The model under review builds one solid part; all positions refer to its coordinate system, in mm. Face numbers are marked on the shaded views. A direction names the side the tool comes from. Coordinates: 2 decimals unless noted, no trailing zeros. Loops run counter-clockwise (first coordinate to the right, second up) from the corner with the lowest first, then second, coordinate; pieces in that order, holes last. Notation, with made-up numbers: (72, -1) - (100, -1) arc R10 cw to (100, 6) - close; hole circle Ø1 at (-1, 84). An arc over 180 degrees is marked (long way). One line per item, written item: value. Start each with the question number.
1. Insertion check: P1, Ø4, axis at x = 45.5, z = 23, coming from the +Y side; P2, Ø1.3, axis at y = 15, z = 20, coming from the -X side; P3, Ø1.3, axis at x = 66, z = 38, coming from the +Y side. Each pin has a flat end and moves straight along its axis. Give the tip position at first contact, or say it passes through.
2. We need section D-D, the plane x = 37. Give the boundary of the cut face in (y, z) (3 decimals), then the cut area to 3 significant figures.
3. To check wall thickness, follow line 1 (Y direction, x = 71.55, z = 26.25); line 2 (Y direction, x = 71.9, z = 19.25) (3 decimals); line 3 (Y direction, x = 58.5, z = 29.5). State the ranges of each line that lie inside material, in increasing order.
4. We need section A-A, the plane z = 19.25. Count the separate pieces of the cut face and the enclosed holes in it, then the cut area to 3 significant figures.
5. For the marked faces 1 and 2, list the 3-axis set-ups (+Z, -Z, +X, -X, +Y, -Y) from which the entire face can be reached by the end or side of a thin tool; tool diameter is ignored.
6. Mouldability with a two-part tool opening along X and no side actions: class the marked faces 3, 4, 5 and 6 as +X half, -X half, draft (parallel to the pull), parting line (faces both ways), or undercut.
7. We need section B-B, the plane y = 61.5. Give the boundary of the cut face in (x, z), then the cut area to 3 significant figures.
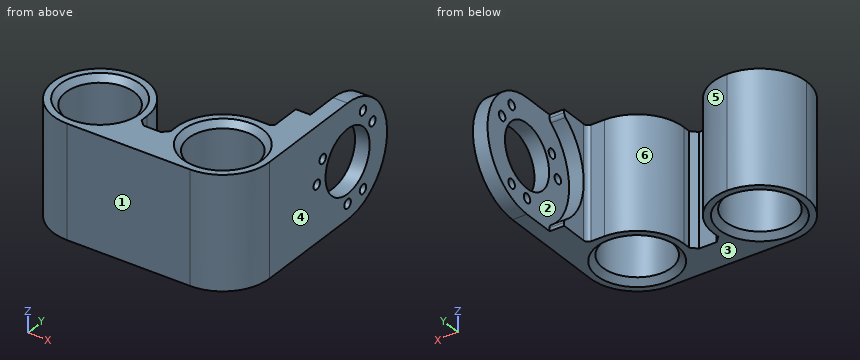
from build123d import *

# Parameters (mm, degrees)
SKETCH1_W               = 74
SKETCH1_H               = 32
SKETCH1_R               = 11.725
BOSS_EXTRUDE1_DEPTH     = 38.5
SKETCH2_R               = 1.575
SKETCH2_R_2             = 10.75
BOSS_EXTRUDE2_DEPTH     = 5
BOSS_EXTRUDE3_DEPTH     = 5
CUT_EXTRUDE1_DEPTH      = 112.012668196
CUT_EXTRUDE1_DEPTH_BACK = 112.012668196
SKETCH4_W               = 10
SKETCH4_H               = 25
SKETCH4_H_2             = 4.450035805
CUT_EXTRUDE2_DEPTH      = 104.814669361
CUT_EXTRUDE2_DEPTH_BACK = 8
SKETCH5_R               = 1.525
FILLET8_R               = 16
FILLET9_R               = 1.5
FILLET10_SIZE           = 2


with BuildPart() as part:
    # Sketch1 → Boss-Extrude1 (new body)
    with BuildSketch(Plane.XY):
        with Locations((37, 16)):
            Rectangle(SKETCH1_W, SKETCH1_H)
        with Locations((16, 16)):
            Circle(SKETCH1_R, mode=Mode.SUBTRACT)
        with Locations((58, 16)):
            Circle(SKETCH1_R, mode=Mode.SUBTRACT)
    extrude(amount=BOSS_EXTRUDE1_DEPTH)

    # Sketch2 → Boss-Extrude2 (add)
    with BuildSketch(Plane(origin=(74, 0, 0), x_dir=(0, 0, -1), z_dir=(1, 0, 0))):
        with BuildLine():
            Line((-38.5, 32), (0, 32))
            Line((0, 32), (0, 54))
            ThreePointArc((0, 54), (-19.25, 73.25), (-38.5, 54))
            Line((-38.5, 54), (-38.5, 32))
        make_face()
        with Locations((-6.259618943, 61.5)):
            Circle(SKETCH2_R, mode=Mode.SUBTRACT)
        with Locations((-26.25, 41.875644347)):
            Circle(SKETCH2_R, mode=Mode.SUBTRACT)
        with Locations((-32.240381057, 61.5)):
            Circle(SKETCH2_R, mode=Mode.SUBTRACT)
        with Locations((-26.25, 66.124355653)):
            Circle(SKETCH2_R, mode=Mode.SUBTRACT)
        with Locations((-19.25, 39)):
            Circle(SKETCH2_R, mode=Mode.SUBTRACT)
        with Locations((-19.25, 54)):
            Circle(SKETCH2_R_2, mode=Mode.SUBTRACT)
        with Locations((-5.25, 54)):
            Circle(SKETCH2_R, mode=Mode.SUBTRACT)
    extrude(amount=-BOSS_EXTRUDE2_DEPTH)

    # Sketch3 → Boss-Extrude3 (add)
    with BuildSketch(Plane.ZY.offset(-69)):
        with BuildLine():
            Line((0, 43), (0, 32))
            Line((0, 32), (38.5, 32))
            Line((38.5, 32), (38.5, 43))
            Line((38.5, 43), (36.548843892, 43))
            ThreePointArc((36.548843892, 43), (19.25, 33.5), (1.951156108, 43))
            Line((1.951156108, 43), (0, 43))
        make_face()
    extrude(amount=BOSS_EXTRUDE3_DEPTH)

    # Sketch4 → Cut-Extrude1 (cut, two sides: drawn at the far end of the back side and taken through both)
    with BuildSketch(Plane(origin=(0, 0, 0), x_dir=(-1, 0, 0), z_dir=(0, 0, -1)).offset(-CUT_EXTRUDE1_DEPTH_BACK)):
        with Locations((-37, 23.950035805)):
            Rectangle(SKETCH4_W, SKETCH4_H)
        with Locations((-37, 34.225017902)):
            Rectangle(SKETCH4_W, SKETCH4_H_2)
    extrude(amount=CUT_EXTRUDE1_DEPTH + CUT_EXTRUDE1_DEPTH_BACK, mode=Mode.SUBTRACT)

    # Sketch5 → Cut-Extrude2 (cut, two sides: drawn at the far end of the back side and taken through both)
    with BuildSketch(Plane(origin=(0, 11.450035805, 0), x_dir=(1, 0, 0), z_dir=(0, 1, 0)).offset(-CUT_EXTRUDE2_DEPTH_BACK)):
        with Locations(Location((37, -19.25, 0), (0, 0, 90))):
            Circle(SKETCH5_R)
    extrude(amount=CUT_EXTRUDE2_DEPTH + CUT_EXTRUDE2_DEPTH_BACK, mode=Mode.SUBTRACT)

    # Fillet8
    fillet8_edges = [part.edges().sort_by_distance(p)[0] for p in [
        (42, 32, 19.25),
        (32, 32, 19.25),
        (0, 32, 19.25),
        (0, 0, 19.25),
        (74, 0, 19.25),
    ]]
    fillet(fillet8_edges, radius=FILLET8_R - 0.0001)  # a hair under: the kernel refuses the full size

    # Fillet9
    fillet9_edges = [part.edges().sort_by_distance(p)[0] for p in [
        (66.5, 43, 36.548843892),
        (66.5, 43, 1.951156108),
        (64, 32, 19.25),
    ]]
    fillet(fillet9_edges, radius=FILLET9_R - 0.0001)  # a hair under: the kernel refuses the full size

    # Fillet10
    fillet10_edges = [part.edges().sort_by_distance(p)[0] for p in [
        (4.275, 16, 0),
        (4.275, 16, 38.5),
        (46.275, 16, 0),
        (46.275, 16, 38.5),
        (42, 11.450035805, 19.25),
        (32, 11.450035805, 19.25),
    ]]
    chamfer(fillet10_edges, length=FILLET10_SIZE)


solid = part.part
Findings below:
1. P1: y = 28.07
1. P2: x = 0
1. P3: y = 43
2. outline: (0, 0) - (11.45, 0) - (11.45, 17.725) - (3.45, 17.725) - (3.45, 20.775) - (11.45, 20.775) - (11.45, 38.5) - (0, 38.5) - close
2. area: 416 mm2
3. line 1: 7.49 to 40.3, 43.45 to 45.84, 62.16 to 64.55, 67.7 to 71.93
3. line 2: 8.076 to 37.425, 40.575 to 43.25, 64.75 to 73.25
3. line 3: 0.01 to 4.29, 27.71 to 32
4. separate pieces: 3
4. enclosed holes: 2
4. area: 1,090 mm2
5. face 1: +Z, -Z, +X, -X, -Y
5. face 2: -X, +Y
6. face 3: draft
6. face 4: +X half
6. face 5: undercut
6. face 6: undercut
7. outline: (69, 1.52) - (74, 1.52) - (74, 4.68) - (69, 4.68) - close; (69, 7.83) - (74, 7.83) - (74, 11.55) - (69, 11.55) - close; (69, 26.95) - (74, 26.95) - (74, 30.67) - (69, 30.67) - close; (69, 33.82) - (74, 33.82) - (74, 36.98) - (69, 36.98) - close
7. area: 68.8 mm2
